Read the model definition and answer for the solid it produces. Units are mm, in the model's axes. Face numbers are marked on the shaded views. Coordinates: 2 decimals unless noted, no trailing zeros. Use one line per item in the form item = value. Start each with the question number.
1. Find the intervals of material crossed by probe 1 along Z at (x, y) = (2.85, 0); probe 2 along Y at (x, z) = (2.9, 0); probe 3 along Z at (x, y) = (3.7, -4.25), in increasing order. Write a range as [from, to].
2. For a pull along Y with two mould halves and no side action, classify the marked faces 1, 2 and 3 as released by +Y, released by -Y, zero draft, split by the parting line, or undercut.
3. Flat-ended cylindrical pins translate along their axes: pin 1 (2 mm diameter, centred on x = 1.5, y = 0, fed in from -Z); pin 2 (1 mm diameter, centred on x = 2, z = -4, fed in from -Y); pin 3 (2 mm diameter, centred on x = 3.5, z = 4.5, fed in from -Y). Find the tip coordinate at first contact, or state that the pin passes through.
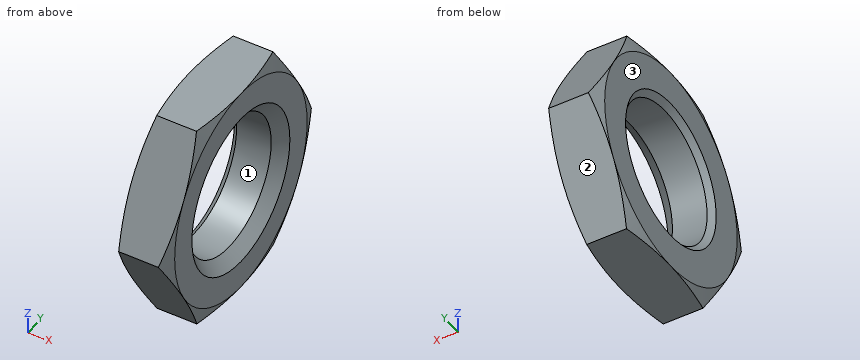
from build123d import *

# Parameters (mm, degrees)
RESSALTO_EXTRUS_O1_DEPTH = 4.6
CHANFRO1_SIZE            = 0.5
ESBO_O8_OUTSIDE_W        = 98.338
ESBO_O8_OUTSIDE_H        = 101.254
ESBO_O8_OUTSIDE_R        = 9.5
CORTE_EXTRUS_O1_DEPTH    = 13
CORTE_EXTRUS_O1_DRAFT    = -70
ESBO_O9_OUTSIDE_W        = 98.338
ESBO_O9_OUTSIDE_H        = 101.254
ESBO_O9_OUTSIDE_R        = 9.5
CORTE_EXTRUS_O2_DEPTH    = 13
CORTE_EXTRUS_O2_DRAFT    = -70


with BuildPart() as part:
    # Esboço1 → Ressalto-extrusão1 (new body)
    with BuildSketch(Plane(origin=(0, 0, 0), x_dir=(0, 0, -1), z_dir=(1, 0, 0))):
        Polygon((9.487887431, 5.505753848), (-0.024178983, 10.969628467), (-9.512066414, 5.46387462), (-9.487887431, -5.505753848), (0.024178983, -10.969628467), (9.512066414, -5.46387462), align=None)
    extrude(amount=RESSALTO_EXTRUS_O1_DEPTH)

    # Esboço6 → Furo roscado de M141 (revolve, cut)
    with BuildSketch(Plane(origin=(4.6, 0, 0), x_dir=(0, 0, -1), z_dir=(0, 1, 0))):
        Polygon((0, 0), (0, 4.6), (6, 4.6), (6, 1.025), (7.025, 0), align=None)
    revolve(axis=Axis((10.95, 0, 0), (-1, 0, 0)), mode=Mode.SUBTRACT)

    # Chanfro1
    chanfro1_edges = [part.edges().sort_by_distance(p)[0] for p in [
        (0, 0, 6),
    ]]
    chamfer(chanfro1_edges, length=CHANFRO1_SIZE)


with BuildPart() as corte_extrus_o1_tool:
    # Esboço8 outside → Corte-extrusão1 (with draft: the straight prism first)
    with BuildSketch(Plane.ZY):
        Rectangle(ESBO_O8_OUTSIDE_W, ESBO_O8_OUTSIDE_H)
        Circle(ESBO_O8_OUTSIDE_R, mode=Mode.SUBTRACT)
    extrude(amount=-CORTE_EXTRUS_O1_DEPTH)
    # Corte-extrusão1: the draft: its side faces are tilted about the plane it starts from
    corte_extrus_o1_sides = [corte_extrus_o1_tool.faces().sort_by_distance(p)[0] for p in [
        (6.5, -50.627, 0),
        (6.5, 0, 49.169),
        (6.5, 50.627, 0),
        (6.5, 0, -49.169),
        (6.5, 0, -9.5),
    ]]
    draft(corte_extrus_o1_sides, Plane.ZY, CORTE_EXTRUS_O1_DRAFT)


with BuildPart() as part_1:
    add(part.part)

    # Corte-extrusão1: cut by corte_extrus_o1_tool
    add(corte_extrus_o1_tool.part, mode=Mode.SUBTRACT)


with BuildPart() as corte_extrus_o2_tool:
    # Esboço9 outside → Corte-extrusão2 (with draft: the straight prism first)
    with BuildSketch(Plane(origin=(4.6, 0, 0), x_dir=(0, 0, -1), z_dir=(1, 0, 0))):
        Rectangle(ESBO_O9_OUTSIDE_W, ESBO_O9_OUTSIDE_H)
        Circle(ESBO_O9_OUTSIDE_R, mode=Mode.SUBTRACT)
    extrude(amount=-CORTE_EXTRUS_O2_DEPTH)
    # Corte-extrusão2: the draft: its side faces are tilted about the plane it starts from
    corte_extrus_o2_sides = [corte_extrus_o2_tool.faces().sort_by_distance(p)[0] for p in [
        (-1.9, -50.627, 0),
        (-1.9, 0, -49.169),
        (-1.9, 50.627, 0),
        (-1.9, 0, 49.169),
        (-1.9, 0, 9.5),
    ]]
    draft(corte_extrus_o2_sides, Plane(origin=(4.6, 0, 0), x_dir=(0, 0, -1), z_dir=(1, 0, 0)), CORTE_EXTRUS_O2_DRAFT)


with BuildPart() as part_2:
    add(part_1.part)

    # Corte-extrusão2: cut by corte_extrus_o2_tool
    add(corte_extrus_o2_tool.part, mode=Mode.SUBTRACT)


solid = part_2.part
Computed values:
q1.probe_1 = [-9.5, -6], [6, 9.5]
q1.probe_2 = [-10.96, -6], [6, 10.96]
q1.probe_3 = [-9.51, -4.41], [4.41, 9.49]
q2.face_1 = undercut
q2.face_2 = released by +Y
q2.face_3 = zero draft
q3.pin_1 = -9.5
q3.pin_2 = -8.95
q3.pin_3 = -8.95
